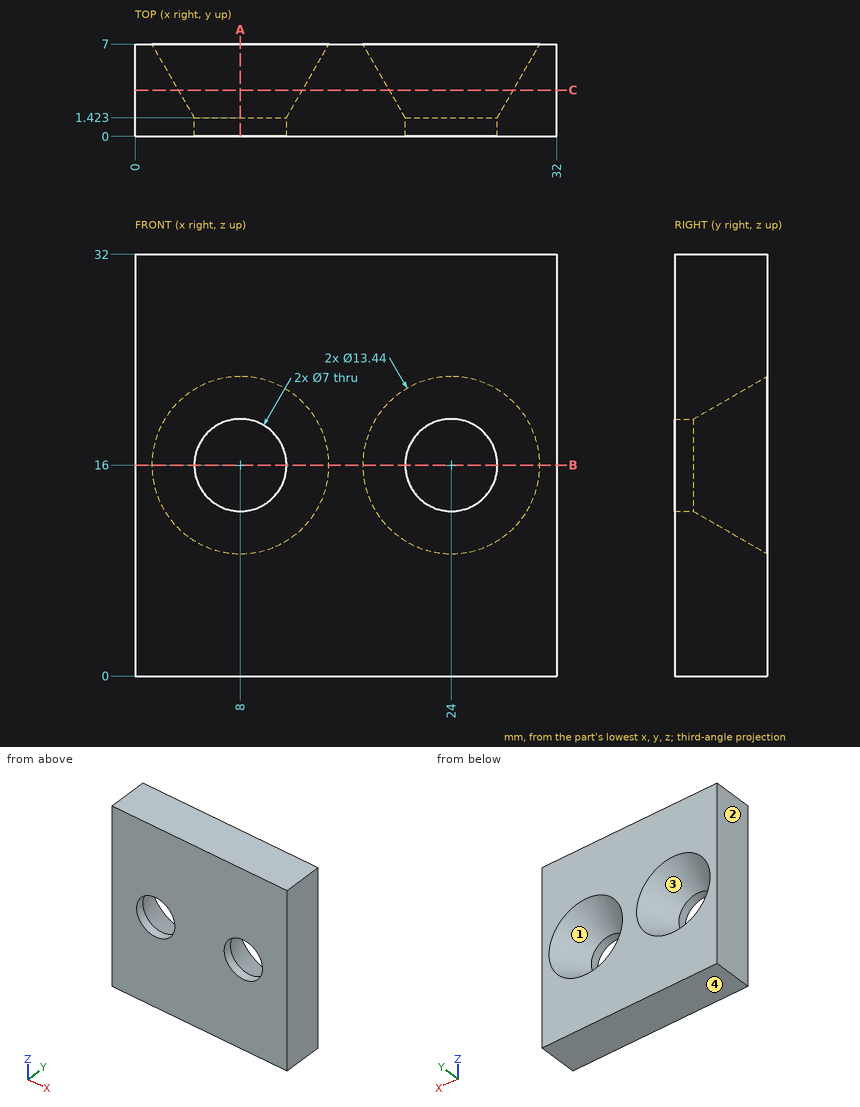
The drawing under review shows one solid part. Ordinate dimensions are in mm from its lowest x, y, z. Give positions to 0.01 mm unless a question says otherwise; leave off trailing zeros. Loops run counter-clockwise (first coordinate to the right, second up) from the corner with the lowest first, then second, coordinate; pieces in that order, holes last. Notation, with made-up numbers: M 34.25,40.25 L 59.25,40.25 A25 ccw 59.25,74.25 Z; hole C 54.5,-38 d6. An arc over 180 degrees is marked long. Return JSON: item names as keys, results as strings. Group by question number.
Item 1: For probe 1 along X at (y, z) = (0.95, 16); probe 2 along X at (y, z) = (2.75, 18); probe 3 along Z at (x, y) = (12, 4.25) (1 decimal), list the stretches that pass through material, from the lowest coordinate up.
Item 2: Insertion check: pin 1 Ø6.5 at (x, z) = (24, 16) entering from -Y. The pin has a flat end and moves straight along its axis. Give the tip position at first contact, or say it passes through.
Item 3: We need section A-A (x = 8). Give the boundary of the cut face in (y, z), and give its area (3 significant figures).
Item 4: We need section C-C (y = 3.5). Give the boundary of the cut face in (x, z).
Item 5: Mouldability with a two-part tool opening along X and no side actions: class the marked faces 1, 2, 3 and 4 as released by +X, released by -X, zero draft, split by the parting line, or undercut.
Item 6: We need section B-B (z = 16). Give the boundary of the cut face in (x, y), and give its area (3 significant figures).
Output:
{
 "1": {"probe 1": "x = 0 to 4.5, 11.5 to 20.5, 27.5 to 32", "probe 2": "x = 0 to 4.23, 11.77 to 20.23, 27.77 to 32", "probe 3": "z = 0 to 12.8, 19.2 to 32"},
 "2": {"pin 1": "passes through"},
 "3": {"outline": "M 0,0 L 7,0 L 7,9.28 L 1.42,12.5 L 0,12.5 Z; M 0,19.5 L 1.42,19.5 L 7,22.72 L 7,32 L 0,32 Z", "area": "157 mm^2"},
 "4": {"outline": "M 0,0 L 32,0 L 32,32 L 0,32 Z; hole C 8,16 d9.4; hole C 24,16 d9.4"},
 "5": {"face 1": "undercut", "face 2": "released by -X", "face 3": "undercut", "face 4": "zero draft"},
 "6": {"outline": "M 0,0 L 4.5,0 L 4.5,1.42 L 1.28,7 L 0,7 Z; M 11.5,0 L 20.5,0 L 20.5,1.42 L 17.28,7 L 14.72,7 L 11.5,1.42 Z; M 27.5,0 L 32,0 L 32,7 L 30.72,7 L 27.5,1.42 Z", "area": "90.1 mm^2"}
}
